The model under review builds one solid part; all positions refer to its coordinate system, in mm. A direction names the side the tool comes from. Give positions to 0.01 mm unless a question says otherwise; leave off trailing zeros. Loops run counter-clockwise (first coordinate to the right, second up) from the corner with the lowest first, then second, coordinate; pieces in that order, holes last. Notation, with made-up numbers: M -31,30.5 L 15,30.5 A31 cw 15,65.5 Z; hole C -40,66.25 d11. An arc over 180 degrees is marked long. Return JSON: item names as keys, results as strings. Group by question number.
```python
from build123d import *

# Parameters (mm, degrees)
F0_W      = 9
F0_H      = 9
F1_DEPTH  = 12
F3_DEPTH  = 5
F4_R      = 4
F5_DEPTH  = 5
F7_DEPTH  = 4
F8_R      = 3
F9_DEPTH  = 5
F10_W     = 0.5
F10_H     = 0.2
F11_DEPTH = 5
F12_SIZE  = 0.5


with BuildPart() as f1:
    # F0 (on Top) → F1 (new body)
    with BuildSketch(Plane.XY):
        Rectangle(F0_W, F0_H)
    extrude(amount=F1_DEPTH)

    # F2 (on face) → F3 (join)
    with BuildSketch(Plane.XY.offset(12)):
        with BuildLine():
            ThreePointArc((0, -4.5), (3.1819805153, -3.1819805153), (4.5, 0))
            ThreePointArc((4.5, 0), (3.1819805153, 3.1819805153), (0, 4.5))
            ThreePointArc((0, 4.5), (-3.1819805153, 3.1819805153), (-4.5, 0))
            ThreePointArc((-4.5, 0), (-3.1819805153, -3.1819805153), (0, -4.5))
        make_face()
    extrude(amount=F3_DEPTH)

    # F4 (on face) → F5 (join)
    with BuildSketch(Plane.XY.offset(17)):
        Circle(F4_R)
    extrude(amount=F5_DEPTH)

    # F6 (on face) → F7 (cut)
    with BuildSketch(Plane.XY.offset(22)):
        with BuildLine():
            Line((-2.5, 1.5), (-3.7080992435, 1.5))
            ThreePointArc((-3.7080992435, 1.5), (-4, 0), (-3.7080992435, -1.5))
            Line((-3.7080992435, -1.5), (-2.5, -1.5))
            Line((-2.5, -1.5), (-2.5, 1.5))
        make_face()
        with BuildLine():
            ThreePointArc((3.7080992435, -1.5), (3.92634671, -0.7640690498), (4, 0))
            ThreePointArc((4, 0), (3.92634671, 0.7640690498), (3.7080992435, 1.5))
            Line((3.7080992435, 1.5), (2.5, 1.5))
            Line((2.5, 1.5), (2.5, -1.5))
            Line((2.5, -1.5), (3.7080992435, -1.5))
        make_face()
    extrude(amount=-F7_DEPTH, mode=Mode.SUBTRACT)

    # F8 (on face) → F9 (join)
    with BuildSketch(Plane.XY.offset(22)):
        Circle(F8_R)
    extrude(amount=F9_DEPTH)

    # F10 (on face) → F11 (join)
    with BuildSketch(Plane.YZ.offset(4.5)):
        with Locations((-3, 8.5)):
            Rectangle(F10_W, F10_H)
        with Locations((0, 8.5)):
            Rectangle(F10_W, F10_H)
        with Locations((3, 8.5)):
            Rectangle(F10_W, F10_H)
        with Locations((-3, 3.5)):
            Rectangle(F10_W, F10_H)
        with Locations((0, 3.5)):
            Rectangle(F10_W, F10_H)
        with Locations((3, 3.5)):
            Rectangle(F10_W, F10_H)
    extrude(amount=F11_DEPTH)

    # F12
    f12_edges = [f1.edges().sort_by_distance(p)[0] for p in [
        (-3, 0, 27),
        (0, 4, 22),
        (0, -4, 22),
    ]]
    chamfer(f12_edges, length=F12_SIZE)


solid = f1.part
```
(1) For probe 1 along Z at (x, y) = (7, 0); probe 2 along X at (y, z) = (-1.25, 2.25); probe 3 along Z at (x, y) = (4.25, 2), list the stretches that pass through material, from the lowest coordinate up.
(2) For pin 1 (0.6 mm diameter, centred on x = 6.5, y = 0, fed in from -Z); pin 2 (0.6 mm diameter, centred on x = 3, z = 20, fed in from +Y); pin 3 (3.5 mm diameter, centred on y = 0, z = 19.5, fed in from +X); pin 4 (3 mm diameter, centred on x = 6.5, z = 14.5, fed in from -Y), all flat-tipped, find the tip position at first contact; note any pin that passes through.
(3) Add section A-A (x = 7). Write out the cut boundary in (y, z).
(4) Add section D-D (z = 14.75). Write out the cut boundary in (x, y).
(5) For faces 1 (the flat face through (4, -4, 12)), 2 (the flat face through (-2.5, 0, 20)), 3 (the flat face through (3, 0, 18)), 4 (the flat face through (-3, -3, 17)), list the 3-axis set-ups (+Z, -Z, +X, -X, +Y, -Y) from which the entire face can be reached by the end or side of a thin tool; tool diameter is ignored.
(6) Add section C-C (z = 23.75). Write out the cut boundary in (x, y), and give its area (3 significant figures).
(7) Mouldability with a two-part tool opening along Z and no side actions: class faces 5 (the flat face through (2.5, 0, 20)), 6 (the flat face through (-4, -3, 12)), 7 (the cylindrical face through (-3, 0, 24)) as released by +Z, released by -Z, zero draft, split by the parting line, or undercut.
(8) Add section B-B (z = 11.5). Write out the cut boundary in (x, y).
Verdict:
{
 "1": {"probe 1": "z = 3.4 to 3.6, 8.4 to 8.6", "probe 2": "x = -4.5 to 4.5", "probe 3": "z = 0 to 12"},
 "2": {"pin 1": "stops at z = 3.4", "pin 2": "stops at y = 2.95", "pin 3": "stops at x = 4", "pin 4": "passes through"},
 "3": {"outline": "M -3.25,3.4 L -2.75,3.4 L -2.75,3.6 L -3.25,3.6 Z; M -3.25,8.4 L -2.75,8.4 L -2.75,8.6 L -3.25,8.6 Z; M -0.25,3.4 L 0.25,3.4 L 0.25,3.6 L -0.25,3.6 Z; M -0.25,8.4 L 0.25,8.4 L 0.25,8.6 L -0.25,8.6 Z; M 2.75,3.4 L 3.25,3.4 L 3.25,3.6 L 2.75,3.6 Z; M 2.75,8.4 L 3.25,8.4 L 3.25,8.6 L 2.75,8.6 Z"},
 "4": {"outline": "C 0,0 d9"},
 "5": {"face 1": "+Z, +X, -Y", "face 2": "-X", "face 3": "+X", "face 4": "+Z"},
 "6": {"outline": "C 0,0 d6", "area": "28.3 mm²"},
 "7": {"face 5": "undercut", "face 6": "released by +Z", "face 7": "zero draft"},
 "8": {"outline": "M -4.5,-4.5 L 4.5,-4.5 L 4.5,4.5 L -4.5,4.5 Z"}
}
